Could you check a few things on this drawing? It's one solid part, dimensions in mm from its lowest x, y, z. A direction names the side the tool comes from. Coordinates: 2 decimals unless noted, no trailing zeros. Loops run counter-clockwise (first coordinate to the right, second up) from the corner with the lowest first, then second, coordinate; pieces in that order, holes last.
1) If I drill on line 1 along X through (y, z) = (124, 146); line 2 along Z through (x, y) = (150, 167.5); line 3 along Z through (x, y) = (150, 104), over which ranges is the centre line in solid material (lowest first)?
2) Thinking about a two-plate mould opening in Z: for the marked faces 1, 2, 3 and 4, which applies, released by +Z, released by -Z, zero draft, split by the parting line, or undercut?
3) Imagine slicing it at A-A on x = 150. Please give me the cut outline in (y, z).
4) Imagine slicing it at C-C on y = 232.5. Please give me the cut outline in (x, z).
5) Imagine slicing it at B-B on z = 150. Please give me the cut outline in (x, y), plus the area to 3 significant figures.
6) Imagine slicing it at D-D on x = 203.5. Please give me the cut outline in (y, z) (1 decimal).
7) For the marked faces 5 and 6, which set-ups out of +Z, -Z, +X, -X, +Y, -Y let a thin tool reach every point of the face, with its end or its side?
8) Will these pins go through, and if not, where does the flat tip stop? P1, Ø12, axis at x = 127, y = 277.5, coming from the -Z side; P2, Ø6, axis at x = 173, y = 263.5, coming from the -Z side; P3, Ø12, axis at x = 88.5, y = 215.5, coming from the +Z side; P4, Ø1.5, axis at x = 109.5, z = 438, coming from the +Y side (1 decimal).
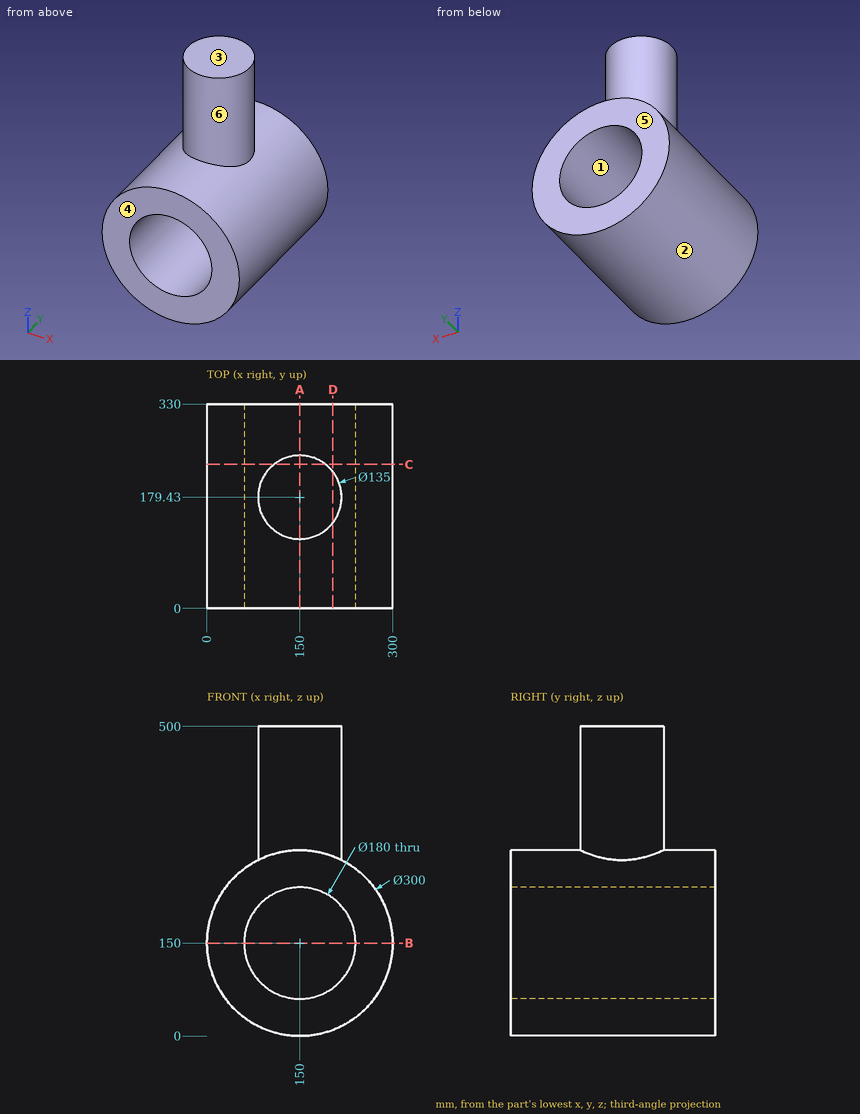
Filled in:
1. line 1: x = 0.05 to 60.09, 239.91 to 299.95
1. line 2: z = 0 to 60, 240 to 500
1. line 3: z = 0 to 60, 240 to 300
2. face 1: undercut
2. face 2: split by the parting line
2. face 3: released by +Z
2. face 4: zero draft
3. outline: (0, 0) - (330, 0) - (330, 60) - (0, 60) - close; (0, 240) - (330, 240) - (330, 300) - (246.93, 300) - (246.93, 500) - (111.93, 500) - (111.93, 300) - (0, 300) - close
4. outline: (108.29, 294.08) arc R150 ccw (long way) to (191.71, 294.08) - (191.71, 500) - (108.29, 500) - close; hole circle Ø180 at (150, 150)
5. outline: (0, 0) - (60, 0) - (60, 330) - (0, 330) - close; (240, 0) - (300, 0) - (300, 330) - (240, 330) - close
5. area: 39,600 mm2
6. outline: (0, 9.9) - (330, 9.9) - (330, 77.6) - (0, 77.6) - close; (0, 222.4) - (330, 222.4) - (330, 290.1) - (220.6, 290.1) - (220.6, 500) - (138.3, 500) - (138.3, 290.1) - (0, 290.1) - close
7. face 5: +Z, -Z, +X, -X, +Y
7. face 6: +Z
8. P1: stops at z = 0.97
8. P2: stops at z = 1.34
8. P3: stops at z = 500
8. P4: stops at y = 234
